Source: CAD feature listing. Evaluate the final solid. Frame: model axes, mm. Face numbers are marked on the shaded views. A direction names the side the tool comes from. Give positions to 0.01 mm unless a question says otherwise; leave off trailing zeros. Write each loop counter-clockwise with the first axis right and the second up, starting at its lowest first coordinate (ties: lowest second). Pieces come first, ordered by that corner, then holes. Notation, with made-up numbers: (77, 57.5) -> (113, 57.5) arc R20 cw to (113, 81.5) -> close; hole circle Ø2 at (-33.5, 13). An arc over 180 degrees is marked (long way). Use one line per item in the form item = value. Start each with the question number.
(1) Cut plane A-A, the plane y = 0. Output: boundary loops of the cut face in (x, z).
(2) Draft query along Z for the marked faces 4, 5 and 6. Return one class per face: pulls with the +Z half, pulls with the -Z half, needs draft (parallel to the pull), parting line crosses it, or undercut.
(3) Cut plane C-C, the plane z = -5.5. Output: boundary loops of the cut face in (x, y).
(4) Cut plane B-B, the plane x = 0.75. Output: boundary loops of the cut face in (y, z), and give its area (3 significant figures).
(5) First-contact query: P1, Ø1.6, axis at x = 5.5, y = -6, coming from the -Z side; P2, Ø2, axis at x = 2.5, y = -7.5, coming from the +Z side; P3, Ø1.5, axis at x = 3.5, y = 6.5, coming from the +Z side. Flat tips, straight axial feed; report the tip coordinate or a pass-through.
(6) Set-up query: the marked faces 1, 2 and 3. Return all of +Z, -Z, +X, -X, +Y, -Y with unobstructed straight access to the full face (end or side cutting, diameter ignored); none if empty.
(7) Material intervals for line 1 along Y through (x, z) = (2.75, 0); line 2 along X through (y, z) = (5.25, -1.25), sorted ascending. Write a range as from..to.
(8) Cut plane D-D, the plane y = 8.5. Output: boundary loops of the cut face in (x, z).
from build123d import *

# Parameters (mm, degrees)
SKETCH1_W               = 6.6
SKETCH1_H               = 6.4
SKETCH2_W               = 3.2
SKETCH2_H               = 5.8
CUT_EXTRUDE1_DEPTH      = 10.5
CUT_EXTRUDE1_DEPTH_BACK = 10.5
SKETCH3_W               = 3.2
SKETCH3_H               = 5.8
CUT_EXTRUDE2_DEPTH      = 10.5
CUT_EXTRUDE2_DEPTH_BACK = 10.5


with BuildPart() as part:
    # Sketch1 → Revolve1 (revolve)
    with BuildSketch(Plane.XY):
        with Locations((3.3, 7.3)):
            Rectangle(SKETCH1_W, SKETCH1_H)
    revolve(axis=Axis((6.6, 0, 0), (-1, 0, 0)))

    # Sketch2 → Cut-Extrude1 (cut, two sides)
    with BuildSketch(Plane.XY) as cut_extrude1_sk:
        with Locations((1.6, 0)):
            Rectangle(SKETCH2_W, SKETCH2_H)
    extrude(amount=CUT_EXTRUDE1_DEPTH, mode=Mode.SUBTRACT)
    extrude(cut_extrude1_sk.sketch, amount=-CUT_EXTRUDE1_DEPTH_BACK, mode=Mode.SUBTRACT)

    # Sketch3 → Cut-Extrude2 (cut, two sides)
    with BuildSketch(Plane(origin=(0, 0, 0), x_dir=(-1, 0, 0), z_dir=(0, 1, 0))) as cut_extrude2_sk:
        with Locations((-5, 0)):
            Rectangle(SKETCH3_W, SKETCH3_H)
    extrude(amount=CUT_EXTRUDE2_DEPTH, mode=Mode.SUBTRACT)
    extrude(cut_extrude2_sk.sketch, amount=-CUT_EXTRUDE2_DEPTH_BACK, mode=Mode.SUBTRACT)


solid = part.part
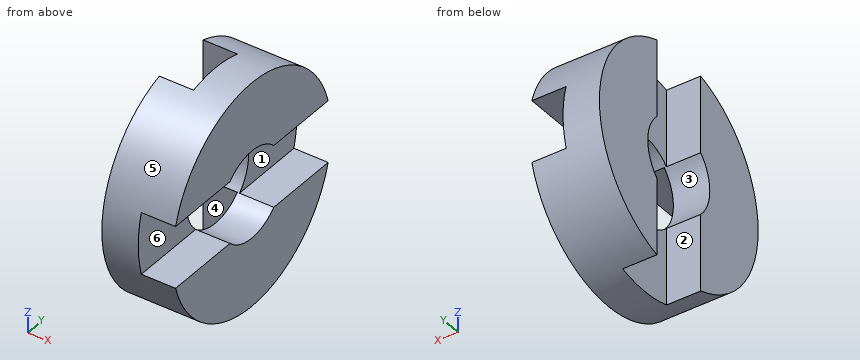
Geometry says:
q1.outline = (3.2, -10.5) -> (6.6, -10.5) -> (6.6, -4.1) -> (3.2, -4.1) -> close; (3.2, 4.1) -> (6.6, 4.1) -> (6.6, 10.5) -> (3.2, 10.5) -> close
q2.face_4 = needs draft
q2.face_5 = parting line crosses it
q2.face_6 = undercut
q3.outline = (0, -8.94) -> (6.6, -8.94) -> (6.6, 8.94) -> (0, 8.94) -> (0, 2.9) -> (3.2, 2.9) -> (3.2, -2.9) -> (0, -2.9) -> close
q4.outline = (-2.9, -10.09) -> (-2.9, -2.9) arc R4.1 cw to (-2.9, 2.9) -> (-2.9, 10.09) arc R10.5 ccw to start; (2.9, -10.09) arc R10.5 ccw to (2.9, 10.09) -> (2.9, 2.9) arc R4.1 cw to (2.9, -2.9) -> close
q4.area = 217 mm^2
q5.P1 = -9.12
q5.P2 = 8.25
q5.P3 = 8.79
q6.face_1 = +X, +Y, -Y
q6.face_2 = +Z, -Z, -X
q6.face_3 = +X, -X
q7.line_1 = -10.5..-4.1, 4.1..10.5
q7.line_2 = 0..3.4
q8.outline = (0, -6.16) -> (6.6, -6.16) -> (6.6, -2.9) -> (3.4, -2.9) -> (3.4, 2.9) -> (6.6, 2.9) -> (6.6, 6.16) -> (0, 6.16) -> close
